from build123d import *

# Parameters (mm, degrees)
SKETCH1_W           = 17.1
SKETCH1_H           = 6
BOSS_EXTRUDE1_DEPTH = 7.7
SKETCH2_W           = 13.5
SKETCH2_H           = 4.6
CUT_EXTRUDE1_DEPTH  = 5
SKETCH3_W           = 1.1
SKETCH3_H           = 6
CUT_EXTRUDE2_DEPTH  = 4.4
SKETCH4_W           = 1.8
SKETCH4_H           = 0.7
CUT_EXTRUDE3_DEPTH  = 5
SKETCH5_W           = 14.9
SKETCH5_H           = 0.9
CUT_EXTRUDE4_DEPTH  = 4.4
SKETCH6_W           = 0.5
SKETCH6_H           = 0.5
BOSS_EXTRUDE2_DEPTH = 3.7


with BuildPart() as part:
    # Sketch1 → Boss-Extrude1 (new body)
    with BuildSketch(Plane(origin=(0, 0, 0), x_dir=(1, 0, 0), z_dir=(0, 1, 0))):
        Rectangle(SKETCH1_W, SKETCH1_H)
    extrude(amount=BOSS_EXTRUDE1_DEPTH)

    # Sketch2 → Cut-Extrude1 (cut)
    with BuildSketch(Plane(origin=(0, 7.7, 0), x_dir=(1, 0, 0), z_dir=(0, 1, 0))):
        Rectangle(SKETCH2_W, SKETCH2_H)
    extrude(amount=-CUT_EXTRUDE1_DEPTH, mode=Mode.SUBTRACT)

    # Sketch3 → Cut-Extrude2 (cut)
    with BuildSketch(Plane(origin=(0, 7.7, 0), x_dir=(1, 0, 0), z_dir=(0, 1, 0))):
        with Locations((-8, 0)):
            Rectangle(SKETCH3_W, SKETCH3_H)
        with Locations((8, 0)):
            Rectangle(SKETCH3_W, SKETCH3_H)
    extrude(amount=-CUT_EXTRUDE2_DEPTH, mode=Mode.SUBTRACT)

    # Sketch4 → Cut-Extrude3 (cut)
    with BuildSketch(Plane(origin=(0, 7.7, 0), x_dir=(1, 0, 0), z_dir=(0, 1, 0))):
        with Locations((-4.6, -2.65)):
            Rectangle(SKETCH4_W, SKETCH4_H)
        with Locations((4.6, -2.65)):
            Rectangle(SKETCH4_W, SKETCH4_H)
    extrude(amount=-CUT_EXTRUDE3_DEPTH, mode=Mode.SUBTRACT)

    # Sketch5 → Cut-Extrude4 (cut)
    with BuildSketch(Plane(origin=(0, 7.7, 0), x_dir=(1, 0, 0), z_dir=(0, 1, 0))):
        with Locations((0, -1.85)):
            Rectangle(SKETCH5_W, SKETCH5_H)
    extrude(amount=-CUT_EXTRUDE4_DEPTH, mode=Mode.SUBTRACT)

    # Sketch6 → Boss-Extrude2 (add)
    with BuildSketch(Plane(origin=(0, 2.7, 0), x_dir=(1, 0, 0), z_dir=(0, 1, 0))):
        with Locations((0, -1.15)):
            Rectangle(SKETCH6_W, SKETCH6_H)
        with Locations((-2.35, -1.15)):
            Rectangle(SKETCH6_W, SKETCH6_H)
        with Locations((2.35, -1.15)):
            Rectangle(SKETCH6_W, SKETCH6_H)
        with Locations((4.7, -1.15)):
            Rectangle(SKETCH6_W, SKETCH6_H)
        with Locations((-4.7, -1.15)):
            Rectangle(SKETCH6_W, SKETCH6_H)
    extrude(amount=BOSS_EXTRUDE2_DEPTH)


solid = part.part
Source: CAD feature listing. Evaluate the final solid. Frame: model axes, mm. A direction names the side the tool comes from. Coordinates: 2 decimals unless noted, no trailing zeros. Write each loop counter-clockwise with the first axis right and the second up, starting at its lowest first coordinate (ties: lowest second). Pieces come first, ordered by that corner, then holes. Notation, with made-up numbers: M 88,46 L 133,46 A20 ccw 133,68 Z; hole C 86,-18 d6. An arc over 180 degrees is marked long. Use a Markdown table: item, result.
1) Reachability of faces 5 (the flat face through (0, 4, 3)), 6 (the flat face through (-7.45, 6, -1)), 7 (the flat face through (7.45, 6, -1)), 8 (the flat face through (-8.55, 2, 0)), 9 (the flat face through (0, 5, -2.3)) from +Z, -Z, +X, -X, +Y, -Y: full face, straight path, thin tool, end or side. Return the list, or none.
Conclusion:
| item | result |
|---|---|
| face 5 | +Z, +X, -X, +Y, -Y |
| face 6 | +Z, -Z, -X, +Y |
| face 7 | +Z, -Z, +X, +Y |
| face 8 | +Z, -Z, -X, +Y, -Y |
| face 9 | +Y |
2) Section D-D, the plane y = 4.25. Give the number of separate pieces and of enclosed holes in the cut face, then the cut area to 3 significant figures.
Conclusion:
| item | result |
|---|---|
| separate pieces | 9 |
| enclosed holes | 0 |
| area | 24.8 mm^2 |
3) Section C-C, the plane x = 3. Output: boundary loops of the cut face in (y, z), then the cut area to 3 significant figures.
Conclusion:
| item | result |
|---|---|
| outline | M 0,-3 L 7.7,-3 L 7.7,-2.3 L 2.7,-2.3 L 2.7,2.3 L 7.7,2.3 L 7.7,3 L 0,3 Z |
| area | 23.2 mm^2 |
4) Section B-B, the plane z = 2.55. Output: boundary loops of the cut face in (x, y), then the cut area to 3 significant figures.
Conclusion:
| item | result |
|---|---|
| outline | M -8.55,0 L 8.55,0 L 8.55,3.3 L 7.45,3.3 L 7.45,7.7 L 5.5,7.7 L 5.5,2.7 L 3.7,2.7 L 3.7,7.7 L -3.7,7.7 L -3.7,2.7 L -5.5,2.7 L -5.5,7.7 L -7.45,7.7 L -7.45,3.3 L -8.55,3.3 Z |
| area | 104 mm^2 |
5) First-contact query: pin 1 Ø0.6 at (x, z) = (0, 1.5) entering from +Y; pin 2 Ø3.5 at (y, z) = (6, 1) entering from -X; pin 3 Ø0.6 at (y, z) = (4.5, 2.5) entering from +X. Flat tips, straight axial feed; report the tip coordinate or a pass-through.
Conclusion:
| item | result |
|---|---|
| pin 1 | stops at y = 6.4 |
| pin 2 | stops at x = -7.45 |
| pin 3 | stops at x = 7.45 |
6) Section A-A, the plane y = 7. Output: boundary loops of the cut face in (x, z), then the cut area to 3 significant figures.
Conclusion:
| item | result |
|---|---|
| outline | M -7.45,-3 L 7.45,-3 L 7.45,1.4 L 6.75,1.4 L 6.75,-2.3 L -6.75,-2.3 L -6.75,1.4 L -7.45,1.4 Z; M -7.45,2.3 L -5.5,2.3 L -5.5,3 L -7.45,3 Z; M -3.7,2.3 L 3.7,2.3 L 3.7,3 L -3.7,3 Z; M 5.5,2.3 L 7.45,2.3 L 7.45,3 L 5.5,3 Z |
| area | 23.5 mm^2 |
7) Ray query, L1, parallel to Z at x = 2.5, y = 3.75; L2, parallel to X at y = 6.25, z = 2.4; L3, parallel to Z at x = -1.5, y = 5.75. Return the intervals inside material, ascending.
Conclusion:
| item | result |
|---|---|
| L1 | z = -3 to -2.3, 0.9 to 1.4, 2.3 to 3 |
| L2 | x = -7.45 to -5.5, -3.7 to 3.7, 5.5 to 7.45 |
| L3 | z = -3 to -2.3, 2.3 to 3 |
8) Mould query, pull axis Z, two halves, no side actions, for faces 1 (the flat face through (0, 4, -3)), 2 (the flat face through (0, 7.7, -2.8)), 3 (the flat face through (-6, 5, 2.3)), 4 (the flat face through (-6.75, 5, 0)). Classes: pulls with the +Z half, pulls with the -Z half, needs draft (parallel to the pull), parting line crosses it, or undercut.
Conclusion:
| item | result |
|---|---|
| face 1 | pulls with the -Z half |
| face 2 | needs draft |
| face 3 | undercut |
| face 4 | undercut |
